Check sheet for the modelled part. Datum: model origin and axes. Units: mm. Round coordinates to 2 decimals unless told otherwise and drop trailing zeros. Order: outer loops, then holes, each group sorted by start corner. A loop starts at its lowest first (then second) coordinate and runs counter-clockwise, first axis right, second up.
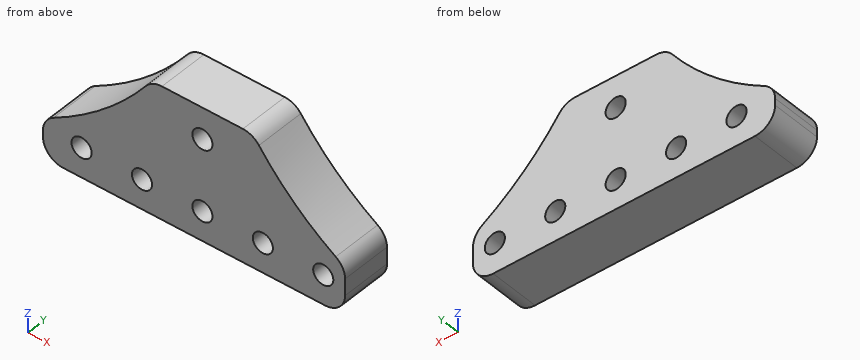
```python
from build123d import *

# Parameters (mm, degrees)
SKETCH1_R           = 1.27
BOSS_EXTRUDE1_DEPTH = 6.35
FILLET1_R           = 2.54


with BuildPart() as part:
    # Sketch1 → Boss-Extrude1 (new body)
    with BuildSketch(Plane(origin=(0, 0, 0), x_dir=(1, 0, 0), z_dir=(0, 1, 0))):
        with BuildLine():
            Line((0, 0), (0, -4.931110589))
            ThreePointArc((0, -4.931110589), (7.586259225, -9.94755683), (13.717235362, -16.665234517))
            Line((13.717235362, -16.665234517), (26.495237193, -16.665234517))
            ThreePointArc((26.495237193, -16.665234517), (31.727577758, -10.741894012), (38.1, -6.06689826))
            Line((38.1, -6.06689826), (38.1, 0))
            Line((38.1, 0), (0, 0))
        make_face()
        with Locations((20.106236278, -12.7)):
            Circle(SKETCH1_R, mode=Mode.SUBTRACT)
        with Locations((4.866236278, -3.72093702)):
            Circle(SKETCH1_R, mode=Mode.SUBTRACT)
        with Locations((12.486236278, -3.72093702)):
            Circle(SKETCH1_R, mode=Mode.SUBTRACT)
        with Locations((20.106236278, -3.72093702)):
            Circle(SKETCH1_R, mode=Mode.SUBTRACT)
        with Locations((27.726236278, -3.72093702)):
            Circle(SKETCH1_R, mode=Mode.SUBTRACT)
        with Locations((35.346236278, -3.72093702)):
            Circle(SKETCH1_R, mode=Mode.SUBTRACT)
    extrude(amount=BOSS_EXTRUDE1_DEPTH)

    # Fillet1
    fillet1_edges = [part.edges().sort_by_distance(p)[0] for p in [
        (13.717235362, 3.175, 16.665234517),
        (0, 3.175, 4.931110589),
        (0, 3.175, 0),
        (38.1, 3.175, 0),
        (38.1, 3.175, 6.06689826),
        (26.495237193, 3.175, 16.665234517),
    ]]
    fillet(fillet1_edges, radius=FILLET1_R)


solid = part.part
```
Item 1: Sectioned sample at A-A (x = 5). Record the cut outline in (y, z), and give its area (3 significant figures).
Answer:
outline: (0, 0) - (6.35, 0) - (6.35, 2.46) - (0, 2.46) - close; (0, 4.98) - (6.35, 4.98) - (6.35, 7.93) - (0, 7.93) - close
area: 34.3 mm2
Item 2: Sectioned sample at B-B (z = 12.7). Record the cut outline in (x, y), and give its area (3 significant figures).
Answer:
outline: (10.47, 0) - (18.84, 0) - (18.84, 6.35) - (10.47, 6.35) - close; (21.38, 0) - (29.74, 0) - (29.74, 6.35) - (21.38, 6.35) - close
area: 106 mm2
Item 3: Go/stop test with flat-tipped pins: P1, Ø1.5, axis at x = 20.11, z = 12.7, coming from the +Y side; P2, Ø2, axis at y = 2.5, z = 13.5, coming from the -X side. Record where each tip stops, or that it passes through.
Answer:
P1: passes through
P2: stops at x = 10.28
Item 4: Scan lines: line 1 along Z through (x, y) = (20, 5.25); line 2 along X through (y, z) = (4, 3.5); line 3 along Z through (x, y) = (9, 4.5). Record each from-to range of solid material in increasing order.
Answer:
line 1: z = 0 to 2.46, 4.99 to 11.43, 13.97 to 16.67
line 2: x = 0 to 3.62, 6.12 to 11.24, 13.74 to 18.86, 21.36 to 26.48, 28.98 to 34.1, 36.6 to 38.1
line 3: z = 0 to 11.22
Item 5: Sectioned sample at C-C (y = 5.75). Record the cut outline in (x, z), and give its area (3 significant figures).
Answer:
outline: (0, 2.54) arc R2.54 ccw to (2.54, 0) - (35.56, 0) arc R2.54 ccw to (38.1, 2.54) - (38.1, 4.64) arc R2.54 ccw to (36.92, 6.78) arc R36.95 cw to (27.23, 15.66) arc R2.54 ccw to (25.21, 16.67) - (15, 16.67) arc R2.54 ccw to (12.98, 15.66) arc R36.95 cw to (1.32, 5.62) arc R2.54 ccw to (0, 3.39) - close; hole circle Ø2.54 at (4.87, 3.72); hole circle Ø2.54 at (12.49, 3.72); hole circle Ø2.54 at (20.11, 3.72); hole circle Ø2.54 at (20.11, 12.7); hole circle Ø2.54 at (27.73, 3.72); hole circle Ø2.54 at (35.35, 3.72)
area: 436 mm2
Item 6: Sectioned sample at D-D (z = 9). Record the cut outline in (x, y), and give its area (3 significant figures).
Answer:
outline: (6.43, 0) - (33.78, 0) - (33.78, 6.35) - (6.43, 6.35) - close
area: 174 mm2
